Part print with two shaded views. Sizes in mm from the minimum x, y, z corner. A direction names the side the tool comes from. Coordinates: 2 decimals unless noted, no trailing zeros. Loops run counter-clockwise (first coordinate to the right, second up) from the corner with the lowest first, then second, coordinate; pieces in that order, holes last. Notation, with made-up numbers: (33, 31.5) -> (60, 31.5) arc R19 cw to (60, 36.5) -> close; hole circle Ø1 at (19.5, 43). An arc over 180 degrees is marked (long way). Return JSON: item names as keys, results as strings. Group by question number.
(1) Saw through at D-D on y = 26.5. Write the cut outline in (x, z).
(2) Saw through at A-A on y = 22.25. Write the cut outline in (x, z).
(3) Saw through at B-B on z = 11.25. Write the cut outline in (x, y).
(4) Saw through at C-C on x = 90. Write the cut outline in (y, z).
(5) Probe L1, parallel to Y at x = 54, z = 7.75; L2, parallel to X at y = 19.5, z = 9; L3, parallel to X at y = 21.25, z = 18.75. List the from-to ranges inside material, lowest first.
(6) Tool access for the marked faces 1 and 2: list every direction of +Z, -Z, +X, -X, +Y, -Y with a clear straight run to the whole face (end or side of a thin tool).
(7) Flat gauge pins, fed straight in: pin 1 Ø4 at (x, z) = (49, 7.5) entering from +Y; pin 2 Ø2 at (x, z) = (15, 17.5) entering from +Y; pin 3 Ø8 at (x, z) = (26, 12.5) entering from +Y. Where does each tip first touch, or does it go through?
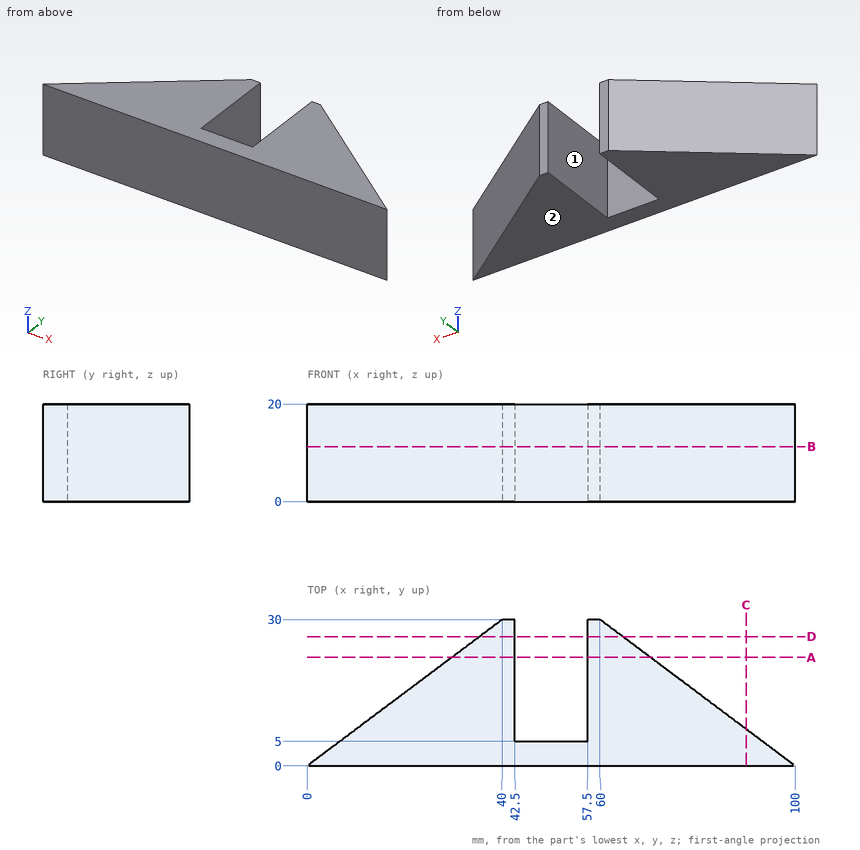
Geometry results:
{
 "1": {"outline": "(35.33, 0) -> (42.5, 0) -> (42.5, 20) -> (35.33, 20) -> close; (57.5, 0) -> (64.67, 0) -> (64.67, 20) -> (57.5, 20) -> close"},
 "2": {"outline": "(29.67, 0) -> (42.5, 0) -> (42.5, 20) -> (29.67, 20) -> close; (57.5, 0) -> (70.33, 0) -> (70.33, 20) -> (57.5, 20) -> close"},
 "3": {"outline": "(0, 0) -> (100, 0) -> (60, 30) -> (57.5, 30) -> (57.5, 5) -> (42.5, 5) -> (42.5, 30) -> (40, 30) -> close"},
 "4": {"outline": "(0, 0) -> (7.5, 0) -> (7.5, 20) -> (0, 20) -> close"},
 "5": {"L1": "0 to 5", "L2": "26 to 42.5, 57.5 to 74", "L3": "28.33 to 42.5, 57.5 to 71.67"},
 "6": {"face 1": "+Z, -Z, +Y", "face 2": "-Z, +X, -X, +Y, -Y"},
 "7": {"pin 1": "y = 5", "pin 2": "y = 12", "pin 3": "y = 22.5"}
}
